Verification items for the finished model (mm, model axes). A direction names the side the tool comes from. Coordinates: 2 decimals unless noted, no trailing zeros. Write each loop counter-clockwise with the first axis right and the second up, starting at its lowest first coordinate (ties: lowest second). Pieces come first, ordered by that corner, then holes. Notation, with made-up numbers: (3, 53) -> (54, 53) arc R16 ccw to (54, 81) -> close; hole circle Ø9 at (-2, 51.5). An arc over 180 degrees is marked (long way). Answer in a Markdown table with one row per item.
```python
from build123d import *

# Parameters (mm, degrees)
F3_D           = 5
F3_CBORE_D     = 8
F3_CBORE_DEPTH = 5


with BuildPart() as f1:
    # F0 (on Front) → F1 (revolve)
    with BuildSketch(Plane.XZ):
        with BuildLine():
            ThreePointArc((25, 40), (39, 26), (25, 12))
            ThreePointArc((25, 12), (11.260843, 8.581576), (0, 0))
            Line((0, 0), (45, 0))
            Line((45, 0), (45, 60))
            Line((45, 60), (15, 60))
            ThreePointArc((15, 60), (5, 50), (15, 40))
            Line((15, 40), (25, 40))
        make_face()
    revolve(axis=Axis((45, 0, 49.649602), (0, 0, -1)))

    # F3 (through all)
    with Locations(Plane.XY.offset(60)):
        with Locations((45, 0)):
            CounterBoreHole(F3_D / 2, F3_CBORE_D / 2, F3_CBORE_DEPTH)


solid = f1.part
```
1. Mould release check, pull along X, two halves, no side actions. Record for faces 1 (the cylindrical face through (42.69, -0.96, 27.11)), 2 (the flat face through (47, 2, 55)), 3 (the flat face through (51, 0, 60)): released by +X, released by -X, zero draft, split by the parting line, or undercut.
Geometry says:
| item | result |
|---|---|
| face 1 | undercut |
| face 2 | undercut |
| face 3 | zero draft |
2. Section check A-A, the plane z = 38.5. Record the boundary of the cut face in (x, y), plus the area to 3 significant figures.
Geometry says:
| item | result |
|---|---|
| outline | circle Ø27.39 at (45, 0); hole circle Ø5 at (45, 0) |
| area | 570 mm^2 |
3. Thickness scan on line 1 (Z direction, x = 57, y = -15); line 2 (Y direction, x = 45, z = 58.9); line 3 (Z direction, x = 45, y = 18.5). Record the ranges inside material, lowest first. Write a range as from..to.
Geometry says:
| item | result |
|---|---|
| line 1 | 0..12.02, 39.98..60 |
| line 2 | -34.56..-4, 4..34.56 |
| line 3 | 0..12.08, 39.92..60 |
4. Section check B-B, the plane z = 19. Record the boundary of the cut face in (x, y), plus the area to 3 significant figures.
Geometry says:
| item | result |
|---|---|
| outline | circle Ø15.75 at (45, 0); hole circle Ø5 at (45, 0) |
| area | 175 mm^2 |
5. Tool access check on faces 4 (the cylindrical face through (41.8, -2.4, 57.5)), 5 (the flat face through (39, -20, 40)), 6 (the flat face through (46, -9, 0)). Record the directions out of +Z, -Z, +X, -X, +Y, -Y that give a thin tool (end or side, any length) a straight path to the whole face; none if there is none.
Geometry says:
| item | result |
|---|---|
| face 4 | +Z |
| face 5 | none |
| face 6 | -Z, +X, -X, +Y, -Y |
6. Depth check by flat-ended pin: P1, Ø7, axis at x = 45, y = 0, coming from the +Z side; P2, Ø12, axis at y = 11, z = 11.5, coming from the +X side; P3, Ø6, axis at y = -10.5, z = 48, coming from the -X side. Enter the tip coordinate at first touch or a pass-through.
Geometry says:
| item | result |
|---|---|
| P1 | z = 55 |
| P2 | x = 82.52 |
| P3 | x = 5.79 |
